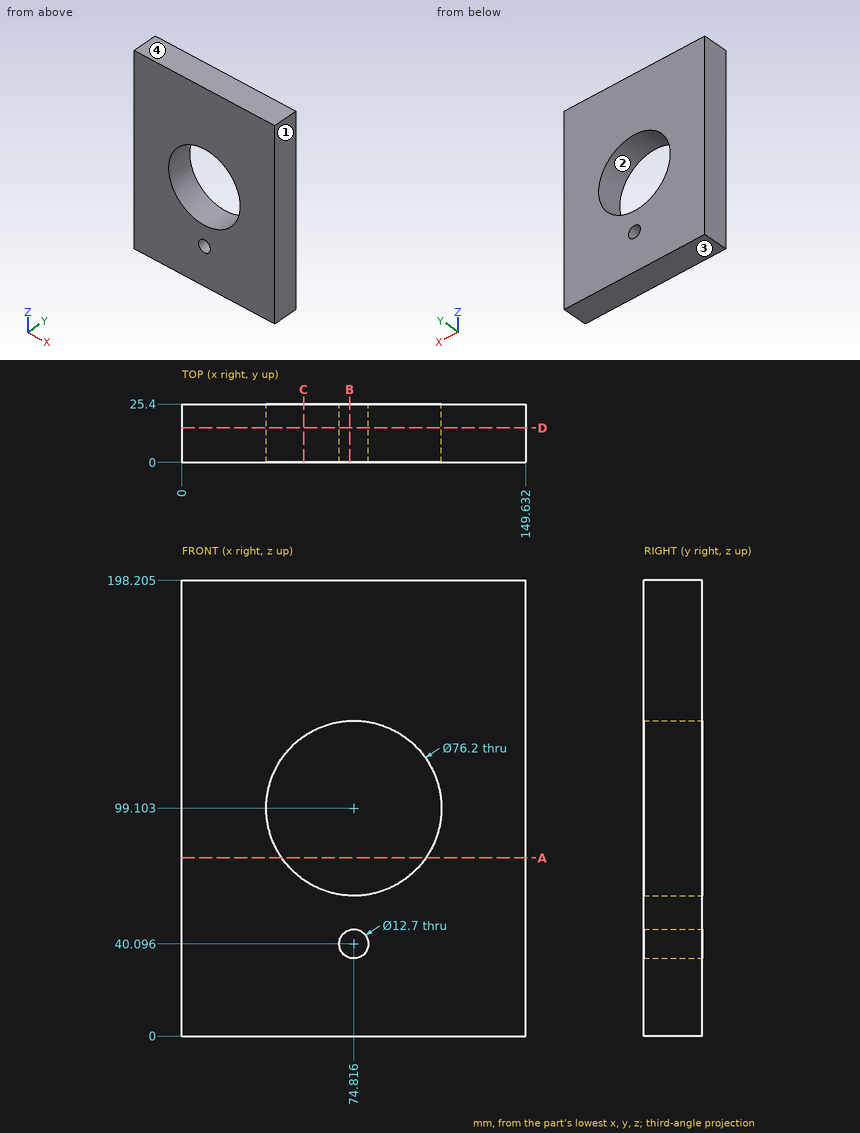
Can you work these out from the drawing? Everything is in mm from the part's minimum corner. Round coordinates to 2 decimals unless told otherwise and drop trailing zeros. Loops run counter-clockwise (first coordinate to the right, second up) from the corner with the lowest first, then second, coordinate; pieces in that order, holes last. Notation, with made-up numbers: (55.25, -24.75) - (108.25, -24.75) arc R13 ccw to (108.25, -2.75) - close; hole circle Ø5 at (-9, 8.25). An arc over 180 degrees is marked (long way). Answer in a Markdown table with one row per item. Add a question column.
(1) If we section it at C-C (x = 53): Please give me the cut outline in (y, z) (1 decimal), plus the area to 3 significant figures.
(2) If we section it at A-A (z = 77.5): Please give me the cut outline in (x, y).
(3) I'm going to push a flat-ended pin straight in: pin 1 (4 mm diameter, centred on y = 7, z = 136, fed in from -X). Where does the tip first touch, or does it pass through?
(4) If we mould it in two halves opening along Z, with no side actions, what happens to the marked faces 1, 2, 3 and 4? For each: pulls with the +Z half, pulls with the -Z half, needs draft (parallel to the pull), parting line crosses it, or undercut.
(5) I need wall thicknesses on line 1 along X through (y, z) = (4.5, 104.5); line 2 along Z through (x, y) = (97, 21) (1 decimal); line 3 along Z through (x, y) = (108.5, 9) (1 decimal). Which ranges of each line are inside material? Lowest first, please.
(6) If we section it at D-D (y = 15): State how many separate pieces and enclosed holes the cut face has, plus the area to 3 significant figures.
(7) If we section it at B-B (x = 73): Please give me the cut outline in (y, z) (1 decimal).
Model answer:
| question | item | result |
|---|---|---|
| 1 | outline | (0, 0) - (25.4, 0) - (25.4, 67.9) - (0, 67.9) - close; (0, 130.3) - (25.4, 130.3) - (25.4, 198.2) - (0, 198.2) - close |
| 1 | area | 3,450 mm² |
| 2 | outline | (0, 0) - (43.43, 0) - (43.43, 25.4) - (0, 25.4) - close; (106.2, 0) - (149.63, 0) - (149.63, 25.4) - (106.2, 25.4) - close |
| 3 | pin 1 | stops at x = 0 |
| 4 | face 1 | needs draft |
| 4 | face 2 | undercut |
| 4 | face 3 | pulls with the -Z half |
| 4 | face 4 | pulls with the +Z half |
| 5 | line 1 | x = 0 to 37.1, 112.53 to 149.63 |
| 5 | line 2 | z = 0 to 68.1, 130.1 to 198.2 |
| 5 | line 3 | z = 0 to 81.3, 116.9 to 198.2 |
| 6 | separate pieces | 1 |
| 6 | enclosed holes | 2 |
| 6 | area | 25,000 mm² |
| 7 | outline | (0, 0) - (25.4, 0) - (25.4, 34) - (0, 34) - close; (0, 46.2) - (25.4, 46.2) - (25.4, 61) - (0, 61) - close; (0, 137.2) - (25.4, 137.2) - (25.4, 198.2) - (0, 198.2) - close |
